Could you check a few things on this model? Use its own coordinates, in mm. Face numbers are marked on the shaded views. A direction names the side the tool comes from. Coordinates: 2 decimals unless noted, no trailing zeros. Write each loop counter-clockwise with the first axis right and the second up, starting at its lowest first coordinate (ties: lowest second). Pieces come first, ordered by that corner, then holes. Notation, with made-up numbers: (33.25, -22) - (88.25, -22) arc R16 cw to (88.25, -12) - close; hole circle Ø1 at (33.5, 75.25). An arc over 180 degrees is marked (long way). Answer as a JSON object with one key per item and string values. Group by question number.
1) On a 3-axis mill with a long thin cutter (end or side, diameter ignored), from which of +Z, -Z, +X, -X, +Y, -Y can I reach the whole of each face in a straight line? I mean the marked faces 1 and 2. Say none if no direction works.
2) Please list where these lines run through material, in increasing order: line 1 along Y through (x, z) = (0, -28); line 2 along Z through (x, y) = (71.5, -30.5); line 3 along Z through (x, y) = (-28, -109).
3) If we section it at D-D (x = 66.5): Write out the boundary of the cut face in (y, z), plus the area to 3 significant figures.
4) We'd pull the mould along Y, two halves only. Please class the marked faces 3, 4 and 5: released by +Y, released by -Y, zero draft, split by the parting line, or undercut.
5) Will these pins go through, and if not, where does the flat tip stop? pin 1 Ø6 at (x, y) = (84, 38) entering from -Z; pin 2 Ø8 at (x, z) = (68.5, -43.5) entering from -Y; pin 3 Ø5 at (x, z) = (33.5, -37.5) entering from +Y.
6) If we section it at A-A (x = 0): Write out the boundary of the cut face in (y, z).
7) If we section it at C-C (z = -27.5): Write out the boundary of the cut face in (x, y), plus the area to 3 significant figures.
8) If we section it at B-B (y = -30.5): Write out the boundary of the cut face in (x, z), plus the area to 3 significant figures.
```python
from build123d import *

# Parameters (mm, degrees)
SKETCH_1_R      = 85
SKETCH_1_R_2    = 52
EXTRUDE_1_DEPTH = 58
SKETCH_2_R      = 120
SKETCH_2_R_2    = 85
EXTRUDE_2_DEPTH = 22
SKETCH_3_R      = 8
EXTRUDE_3_DEPTH = 6


with BuildPart() as part:
    # 草图1 → 凸台-拉伸1 (new body)
    with BuildSketch(Plane.XY):
        Circle(SKETCH_1_R)
        Circle(SKETCH_1_R_2, mode=Mode.SUBTRACT)
    extrude(amount=-EXTRUDE_1_DEPTH)

    # 草图2 → 凸台-拉伸2 (add)
    with BuildSketch(Plane.XY):
        Circle(SKETCH_2_R)
        Circle(SKETCH_2_R_2, mode=Mode.SUBTRACT)
    extrude(amount=-EXTRUDE_2_DEPTH)

    # 草图3 → 凸台-拉伸3 (add)
    with BuildSketch(Plane.XY):
        with Locations((102, 0)):
            Circle(SKETCH_3_R)
        with Locations((51, 88.334591186)):
            Circle(SKETCH_3_R)
        with Locations((-51, 88.334591186)):
            Circle(SKETCH_3_R)
        with Locations((-102, 0)):
            Circle(SKETCH_3_R)
        with Locations((-51, -88.334591186)):
            Circle(SKETCH_3_R)
        with Locations((51, -88.334591186)):
            Circle(SKETCH_3_R)
    extrude(amount=EXTRUDE_3_DEPTH)


solid = part.part
```
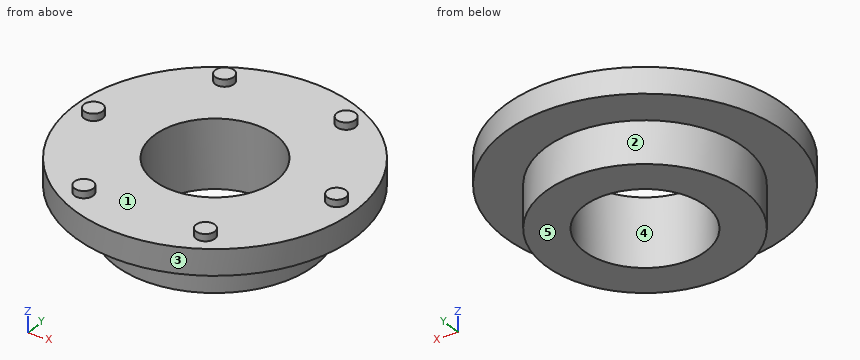
Here are the results:
{
 "1": {"face 1": "+Z", "face 2": "-Z"},
 "2": {"line 1": "y = -85 to -52, 52 to 85", "line 2": "z = -58 to 0", "line 3": "z = -22 to 0"},
 "3": {"outline": "(-99.89, -22) - (-52.94, -22) - (-52.94, -58) - (52.94, -58) - (52.94, -22) - (99.89, -22) - (99.89, 0) - (-99.89, 0) - close", "area": "8,210 mm²"},
 "4": {"face 3": "split by the parting line", "face 4": "undercut", "face 5": "zero draft"},
 "5": {"pin 1": "stops at z = -22", "pin 2": "stops at y = -55.36", "pin 3": "stops at y = 79.15"},
 "6": {"outline": "(-120, -22) - (-85, -22) - (-85, -58) - (-52, -58) - (-52, 0) - (-120, 0) - close; (52, -58) - (85, -58) - (85, -22) - (120, -22) - (120, 0) - (52, 0) - close"},
 "7": {"outline": "circle Ø170 at (0, 0); hole circle Ø104 at (0, 0)", "area": "14,200 mm²"},
 "8": {"outline": "(-116.06, -22) - (-79.34, -22) - (-79.34, -58) - (-42.12, -58) - (-42.12, 0) - (-116.06, 0) - close; (42.12, -58) - (79.34, -58) - (79.34, -22) - (116.06, -22) - (116.06, 0) - (42.12, 0) - close", "area": "5,930 mm²"}
}
